Check sheet for the drawn part. Datum: minimum x, y, z corner. Units: mm. A direction names the side the tool comes from. Round coordinates to 2 decimals unless told otherwise and drop trailing zeros. Loops run counter-clockwise (first coordinate to the right, second up) from the corner with the lowest first, then second, coordinate; pieces in that order, holes last. Notation, with made-up numbers: (89, -4) - (115, -4) arc R27 ccw to (115, 17) - close; hole circle Ø3 at (85, 64.5). An arc over 180 degrees is marked (long way). Use CSV: the item, a comma, the result in double quotes.
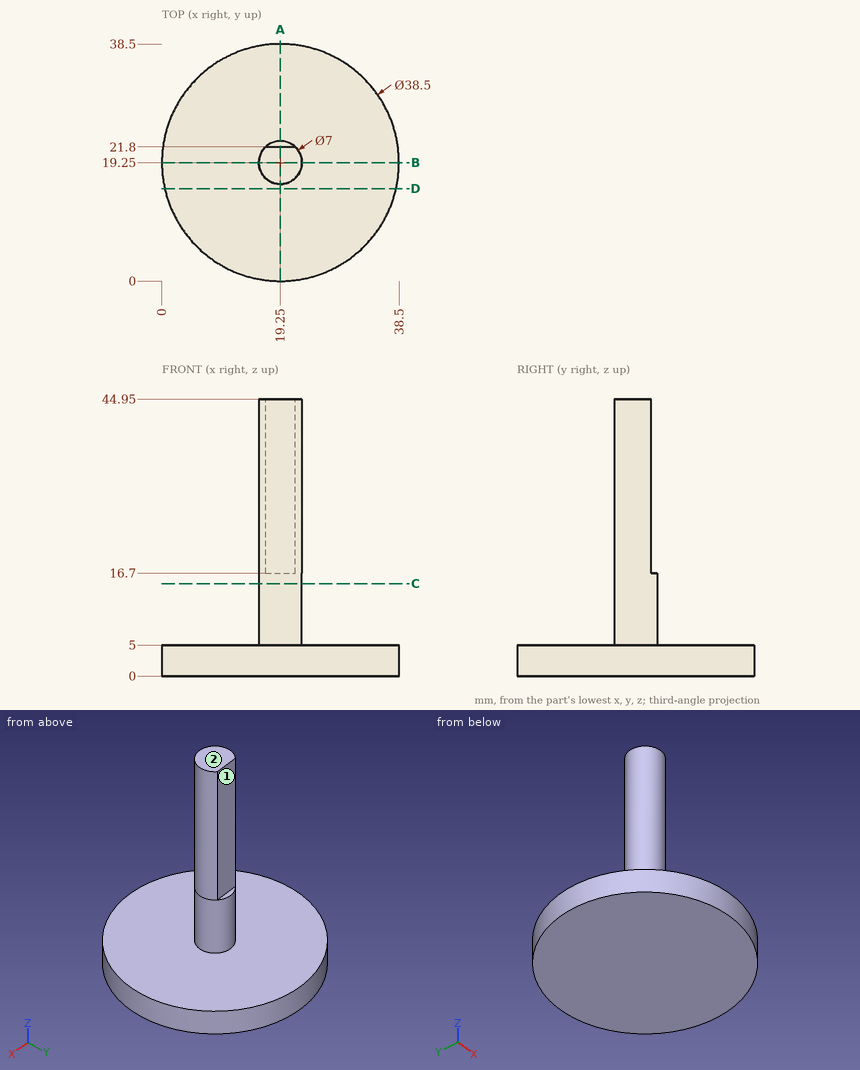
1) Thickness scan on probe 1 along Z at (x, y) = (12, 36.5); probe 2 along X at (y, z) = (21, 14); probe 3 along X at (y, z) = (18.5, 7). Record the ranges inside material, lowest first. Write a range as [from, to].
Returned:
probe 1,"z = [0, 5]"
probe 2,"x = [16.22, 22.28]"
probe 3,"x = [15.83, 22.67]"
2) Cross-section at A-A, the plane x = 19.25. Record the cut outline in (y, z).
Returned:
outline,"(0, 0) - (38.5, 0) - (38.5, 5) - (22.75, 5) - (22.75, 16.7) - (21.8, 16.7) - (21.8, 44.95) - (15.75, 44.95) - (15.75, 5) - (0, 5) - close"
3) Cross-section at B-B, the plane y = 19.25. Record the cut outline in (x, z).
Returned:
outline,"(0, 0) - (38.5, 0) - (38.5, 5) - (22.75, 5) - (22.75, 44.95) - (15.75, 44.95) - (15.75, 5) - (0, 5) - close"
4) Gauge pin test, flat ends, axial feed: pin 1 Ø10 at (y, z) = (17.5, 30) entering from +X; pin 2 Ø2 at (x, y) = (27.5, 25.5) entering from +Z; pin 3 Ø10 at (x, z) = (30.5, 31.5) entering from -Y; pin 4 Ø0.8 at (x, y) = (20.5, 22.5) entering from +Z. Record the tip position at first contact, or that the pin passes through.
Returned:
pin 1,"stops at x = 22.75"
pin 2,"stops at z = 5"
pin 3,"passes through"
pin 4,"stops at z = 16.7"
5) Cross-section at D-D, the plane y = 15. Record the cut outline in (x, z), then the cut area to 3 significant figures.
Returned:
outline,"(0.48, 0) - (38.02, 0) - (38.02, 5) - (0.48, 5) - close"
area,"188 mm²"
6) Cross-section at C-C, the plane z = 15. Record the cut outline in (x, y).
Returned:
outline,"circle Ø7 at (19.25, 19.25)"
7) Access from +Z, -Z, +X, -X, +Y, -Y to the whole of each face (thin tool, end or side, straight path). Record for the marked faces 1 and 2.
Returned:
face 1,"+Z, +X, -X, +Y"
face 2,"+Z, +X, -X, +Y, -Y"
